```python
from build123d import *

# Parameters (mm, degrees)
SKETCH1_R    = 1.5
SHANK_DEPTH  = 8
SKETCH2_R    = 2.75
HEAD_DEPTH   = 3
SOCKET_DEPTH = 1.6


with BuildPart() as part:
    # Sketch1 → Shank (new body)
    with BuildSketch(Plane.XY):
        Circle(SKETCH1_R)
    extrude(amount=SHANK_DEPTH)

    # Sketch2 → Head (add)
    with BuildSketch(Plane.XY.offset(8)):
        Circle(SKETCH2_R)
    extrude(amount=HEAD_DEPTH)

    # Sketch3 → Socket (cut)
    with BuildSketch(Plane.XY.offset(9.4)):
        Polygon((1.443375673, 0), (0.721687836, 1.25), (-0.721687836, 1.25), (-1.443375673, 0), (-0.721687836, -1.25), (0.721687836, -1.25), align=None)
    extrude(amount=SOCKET_DEPTH, mode=Mode.SUBTRACT)


solid = part.part
```
Input: part model. Units: mm. Frame: model coordinates. A direction names the side the tool comes from. Coordinates: 2 decimals unless noted, no trailing zeros. Write each loop counter-clockwise with the first axis right and the second up, starting at its lowest first coordinate (ties: lowest second). Pieces come first, ordered by that corner, then holes. Notation, with made-up numbers: (23.5, -29.5) - (47.5, -29.5) arc R12 ccw to (47.5, -9.5) - close; hole circle Ø8 at (-6.5, 3). An arc over 180 degrees is marked (long way). Put each result on its own line as item: value. Start each with the question number.
1) Cut plane D-D (z = 5). Return the cut outline in (x, y).
2) Mould query, pull axis Y, two halves, no side actions, for faces 1 (the face through (1.088, 0.616, 10.189)), 2 (the face through (1.2, -1.2, 8)), 3 (the face through (-0.596, -2.685, 9.479)). Classes: pulls with the +Y half, pulls with the -Y half, needs draft (parallel to the pull), parting line crosses it, or undercut.
3) Cut plane B-B (x = 0). Return the cut outline in (y, z), plus the area to 3 significant figures.
4) Cut plane A-A (z = 10). Return the cut outline in (x, y).
5) Cut plane C-C (y = -1). Return the cut outline in (x, z), plus the area to 3 significant figures.
6) Contact query for flat-ended pins moving along their axis: pin 1 (1 mm diameter, centred on y = 0.5, z = 9.5, fed in from +X); pin 2 (3 mm diameter, centred on y = -2, z = 2.5, fed in from -X); pin 3 (3 mm diameter, centred on y = -1, z = 4, fed in from +X); pin 4 (1.5 mm diameter, centred on x = 0, z = 1.5, fed in from -Y). Output: stop coordinate, or through.
7) Reachability of faces 4 (the face through (-1.088, -0.616, 10.189)), 5 (the face through (0, 0, 0)), 6 (the face through (-1.5, 0.07, 3.94)) from +Z, -Z, +X, -X, +Y, -Y: full face, straight path, thin tool, end or side. Return the list, or none.
8) Ray query, L1, parallel to Z at x = -1.65, y = -1.25; L2, parallel to Z at x = 0.55, y = 0.05; L3, parallel to X at y = 0.85, z = 9.5. Return the intervals inside material, ascending.
Resolved:
1. outline: circle Ø3 at (0, 0)
2. face 1: undercut
2. face 2: needs draft
2. face 3: parting line crosses it
3. outline: (-2.75, 8) - (-1.5, 8) - (-1.5, 0) - (1.5, 0) - (1.5, 8) - (2.75, 8) - (2.75, 11) - (1.25, 11) - (1.25, 9.4) - (-1.25, 9.4) - (-1.25, 11) - (-2.75, 11) - close
3. area: 36.5 mm2
4. outline: circle Ø5.5 at (0, 0); hole (-1.44, 0) - (-0.72, -1.25) - (0.72, -1.25) - (1.44, 0) - (0.72, 1.25) - (-0.72, 1.25) - close
5. outline: (-2.56, 8) - (-1.12, 8) - (-1.12, 0) - (1.12, 0) - (1.12, 8) - (2.56, 8) - (2.56, 11) - (0.87, 11) - (0.87, 9.4) - (-0.87, 9.4) - (-0.87, 11) - (-2.56, 11) - close
5. area: 30.5 mm2
6. pin 1: stops at x = 2.75
6. pin 2: stops at x = -1.41
6. pin 3: stops at x = 1.5
6. pin 4: stops at y = -1.5
7. face 4: +Z
7. face 5: -Z, +X, -X, +Y, -Y
7. face 6: -Z
8. L1: z = 8 to 11
8. L2: z = 0 to 9.4
8. L3: x = -2.62 to -0.95, 0.95 to 2.62
